The listing builds one solid part. Answer for the finished solid, in the listing's coordinates (mm). A direction names the side the tool comes from. Give positions to 0.01 mm unless a question says otherwise; leave off trailing zeros. Write each loop counter-clockwise with the first axis right and the second up, starting at its lowest first coordinate (ties: lowest second). Pieces come first, ordered by that corner, then holes. Notation, with made-up numbers: (54, 85) -> (65, 85) arc R21 cw to (65, 89) -> close; hole circle Ø2 at (27, 2). An arc over 180 degrees is marked (long way). Put each result on its own line as item: value. Start each with the question number.
1) A cutting plane is placed at D-D (y = 7.75). Write down the section's boundary in (x, z) (3 decimals), then the cut area to 3 significant figures.
2) For faces 4 (the flat face through (-11, 14, 8)), 5 (the flat face through (16.975, 2, -15)), 6 (the flat face through (-21, 26.1, 0)), 7 (the flat face through (26.175, 17, 0)), 8 (the flat face through (27, 5, -5)), determine the directions among +Z, -Z, +X, -X, +Y, -Y from which every point of the face is accessible in a straight line to the end or side of a thin tool.
3) A cutting plane is placed at B-B (y = 18.75). Write down the section's boundary in (x, z) (3 decimals), then the cut area to 3 significant figures.
4) A cutting plane is placed at C-C (z = -19.35). Write down the section's boundary in (x, y) (3 decimals), then the cut area to 3 significant figures.
5) Find the intervals of material crossed by line 1 along X through (y, z) = (2.7, 0) (3 decimals); line 2 along X through (y, z) = (3.1, 4) (3 decimals); line 3 along X through (y, z) = (3.9, -19.35) (3 decimals), in increasing order. Write a range as from..to.
6) For a pull along Y with two mould halves and no side action, classify faces 1 (the flat face through (-12, 5, 2.05)), 2 (the flat face through (39, 26.1, 0)), 3 (the cylindrical face through (22.737, 1.775, -0.347)) as released by +Y, released by -Y, zero draft, split by the parting line, or undercut.
7) A cutting plane is placed at A-A (y = 24.75). Write down the section's boundary in (x, z) (3 decimals), then the cut area to 3 significant figures.
8) Flat-ended cylindrical pins translate along their axes: pin 1 Ø15 at (x, y) = (-8, 12.5) entering from -Z; pin 2 Ø10 at (y, z) = (6.5, 0.5) entering from +X (3 decimals); pin 3 Ø10 at (x, z) = (-13.5, 2) entering from -Y; pin 4 Ø1 at (y, z) = (25, 6) entering from -X. Find the tip coordinate at first contact, or state that the pin passes through.
Autodesk Inventor part; units mm, degrees
ref_plane "YZ Plane" through (0, 0, 0) normal (1, 0, 0) x (0, 1, 0)
ref_plane "XZ Plane" through (0, 0, 0) normal (0, 1, 0) x (-1, 0, 0)
ref_plane "XY Plane" through (0, 0, 0) normal (0, 0, 1) x (1, 0, 0)
sketch "Эскиз1" plane through (0, 0, 0) normal (0, 1, 0) x (-1, 0, 0)
  line L0 (-8.725, 8) -> (8.725, 8)
  line L1 (8.725, 8) -> (8.725, -8)
  line L2 (8.725, -8) -> (-8.725, -8)
  line L3 (-8.725, -8) -> (-8.725, 8)
  line L4 (-8.725, 8) -> (8.725, -8) construction
  line L5 (8.725, 8) -> (-8.725, -8) construction
  point P0 (0, 0)
  dimension "d0" = 17.45
  dimension "d1" = 16
extrude "Выдавливание1" add sketch "Эскиз1" along normal blind 5
sketch "Эскиз2" plane through (-8.725, 0, -8) normal (-1, 0, 0) x (0, 0, 1)
  line L0 (0, 23.1) -> (16, 23.1)
  line L1 (16, 23.1) -> (16, 0)
  line L2 (16, 0) -> (0, 0)
  line L3 (0, 0) -> (0, 23.1)
  line L4 (16, 0) -> (16, 5)
  line L5 (0, 0) -> (0, 5)
  line L6 (0, 0) -> (16, 0)
  line L7 (0, 5) -> (16, 5)
  point P0 (8, 0)
  dimension "d5" = 18.1
extrude "Выдавливание2" add sketch "Эскиз2" along normal blind 5
sketch "Эскиз3" plane through (-8.725, 23.1, 8) normal (0, 1, 0) x (1, 0, 0)
  line L0 (0, 16) -> (-17.5, 16)
  line L1 (-17.5, 16) -> (-17.5, 0)
  line L2 (-17.5, 0) -> (0, 0)
  line L3 (0, 0) -> (0, 16)
  line L4 (0, 0) -> (-5, 0)
  circle A0 centre (-9.5, 8) radius 8
  line L5 (-5, 0) -> (-5, 16)
  point P0 (-9.5, 16)
  point P1 (-9.5, 0)
  point P2 (-5, 8)
  dimension "d49" = 4.5
extrude "Выдавливание3" add sketch "Эскиз3" along normal blind 6 contours L3 L2 L5 A0 L0 | L5 A0 L0 | A0 L5 | A0 L5 | L2 A0 L5
sketch "Эскиз7" plane through (0, 0, 0) normal (0, -1, 0) x (1, 0, 0)
  line L0 (-8.725, -8) -> (-8.725, 8) construction
  line L1 (-8.725, 8) -> (-8.725, -8) construction
  line L2 (-13.725, 8) -> (-13.725, -8) construction
  line L3 (-8.725, -8) -> (-13.725, -8) construction
  line L4 (-13.725, -8) -> (-13.725, 8) construction
  line L5 (-13.725, 8) -> (-8.725, 8) construction
  line L6 (-8.725, 8) -> (-8.725, -8) construction
  line L7 (-13.725, -8) -> (-13.725, 8)
  line L8 (-13.725, 0) -> (-8.725, 0) construction
  line L9 (-11.225, -4) -> (-11.225, 4)
  point P0 (0, 0)
  point P1 (-11.225, 0)
  dimension "d34" = 8
hole "Отверстие3" at (-11.225, 0, -4) at (-11.225, 0, 4) direction (0, 1, 0) diameter 2.2 depth 6
sketch "Эскиз8" plane through (0, 0, 0) normal (0, -1, 0) x (1, 0, 0)
  circle A0 centre (-11.225, -4) radius 1.1
  line L0 (-13.4767, -4) -> (-12.3508, -2.05) construction
  line L1 (-12.3508, -2.05) -> (-10.0992, -2.05)
  line L2 (-10.0992, -2.05) -> (-8.9733, -4)
  line L3 (-8.9733, -4) -> (-10.0992, -5.95)
  line L4 (-10.0992, -5.95) -> (-12.3508, -5.95)
  line L5 (-12.3508, -5.95) -> (-13.4767, -4) construction
  circle A1 centre (-11.225, 4) radius 1.1
  line L6 (-13.4767, 4) -> (-12.3508, 5.95) construction
  line L7 (-12.3508, 5.95) -> (-10.0992, 5.95)
  line L8 (-10.0992, 5.95) -> (-8.9733, 4)
  line L9 (-8.9733, 4) -> (-10.0992, 2.05)
  line L10 (-10.0992, 2.05) -> (-12.3508, 2.05)
  line L11 (-12.3508, 2.05) -> (-13.4767, 4) construction
  line L12 (-13.725, -8) -> (-13.725, 8)
  line L13 (-12.3508, -5.95) -> (-13.725, -5.95)
  line L14 (-13.725, -5.95) -> (-13.725, -2.05)
  line L15 (-13.725, -2.05) -> (-12.3508, -2.05)
  line L16 (-12.3508, -2.05) -> (-12.3508, -5.95) construction
  line L17 (-12.3508, 2.05) -> (-13.725, 2.05)
  line L18 (-13.725, 2.05) -> (-13.725, 5.95)
  line L19 (-13.725, 5.95) -> (-12.3508, 5.95)
  line L20 (-12.3508, 5.95) -> (-12.3508, 2.05) construction
  point P0 (0, 0)
  dimension "d42" = 3.9
extrude "Выдавливание5" cut sketch "Эскиз8" along normal blind 2.1 from surface at -6
sketch "Эскиз4" plane through (-8.725, 23.1, 8) normal (0, -1, 0) x (1, 0, 0)
  arc A0 (-9.5, 0) -> (-9.5, -16) centre (-9.5, -8) ccw
  circle A1 centre (-12.5, -8) radius 4
  arc A2 (-9.5, 0) -> (-9.5, -16) centre (-9.5, -8) ccw
  line L0 (-17.5, -8) -> (-16.5, -8) construction
  line L1 (-16.5, -8) -> (-9.5, -8) construction
  point P0 (8.725, -8)
  dimension "d45" = 8
  dimension "d46" = 1
extrude "Выдавливание6" cut sketch "Эскиз4" against normal blind 3
sketch "Эскиз5" plane through (0, 5, 0) normal (0, 1, 0) x (1, 0, 0)
  line L0 (-8.725, 8) -> (-8.725, -8)
  line L1 (-8.725, 0) -> (-3.725, 0) construction
  point P0 (0, 0)
  dimension "d22" = 5
hole "Отверстие2" at (-3.725, 5, 0) direction (0, -1, 0) diameter 3.2 end through all countersink diameter 6 countersink angle 90
mirror "Зеркальное отражение1" about plane through (8.725, 0, 8) normal (1, 0, 0)
sketch "Эскиз9" plane through (0, 0, 0) normal (0, -1, 0) x (1, 0, 0)
  line L0 (-8.725, 8) -> (26.175, 8) construction
  line L1 (8.725, 8) -> (8.725, -8) construction
  line L2 (-8.725, -8) -> (26.175, -8) construction
  line L3 (2.475, -16.35) -> (14.975, -16.35) construction
  line L4 (14.975, -16.35) -> (14.975, 6.45) construction
  line L5 (14.975, 6.45) -> (2.475, 6.45) construction
  line L6 (2.475, 6.45) -> (2.475, -16.35) construction
  line L7 (2.475, -16.35) -> (14.975, 6.45) construction
  line L8 (14.975, -16.35) -> (2.475, 6.45) construction
  line L9 (16.975, 10.95) -> (0.475, 10.95)
  line L10 (0.475, 10.95) -> (0.475, -22.35)
  line L11 (0.475, -22.35) -> (16.975, -22.35)
  line L12 (16.975, -22.35) -> (16.975, 10.95)
  point P0 (0, 0)
  point P1 (8.725, -4.95)
  point P2 (8.725, 0)
  dimension "d50" = 12.5
  dimension "d51" = 22.8
  dimension "d59" = 4.95
  dimension "d68" = 6
  dimension "d69" = 4.5
  dimension "d70" = 2
  dimension "d71" = 2
extrude "Выдавливание7" add sketch "Эскиз9" against normal up to surface (5 mm away)
sketch "Эскиз10" plane through (0, 5, 0) normal (0, 1, 0) x (1, 0, 0)
  line L0 (2.275, -6.45) -> (15.175, -6.45)
  line L1 (15.175, -6.45) -> (15.175, 16.35)
  line L2 (15.175, 16.35) -> (2.275, 16.35)
  line L3 (2.275, 16.35) -> (2.275, -6.45)
  line L4 (2.275, -6.45) -> (15.175, 16.35) construction
  line L5 (15.175, -6.45) -> (2.275, 16.35) construction
  line L6 (-8.725, 8) -> (0.475, 8)
  line L7 (16.975, -8) -> (0.475, 8) construction
  line L8 (16.975, 8) -> (26.175, 8)
  line L9 (-8.725, -8) -> (0.475, -8)
  line L10 (16.975, 8) -> (0.475, -8) construction
  line L11 (16.975, -8) -> (26.175, -8)
  line L12 (8.725, 0) -> (8.725, 4.95)
  point P0 (0, 0)
  dimension "d54" = 12.9
  dimension "d55" = 22.8
  dimension "d72" = 4.95
extrude "Выдавливание8" cut sketch "Эскиз10" against normal through all
sketch "Эскиз11" plane through (0, 0, 0) normal (0, -1, 0) x (1, 0, 0)
  line L0 (8.725, -22.35) -> (8.725, -16.35) construction
  line L1 (12.725, -19.35) -> (4.725, -19.35)
  line L2 (15.175, -16.35) -> (2.275, -16.35)
  line L3 (0.475, -22.35) -> (16.975, -22.35)
  point P0 (0, 0)
  point P1 (8.725, -19.35)
  dimension "d60" = 8
hole "Отверстие4" at (12.725, 0, -19.35) at (4.725, 0, -19.35) direction (0, 1, 0) diameter 2.2 end through all countersink diameter 4.2 countersink angle 90
sketch "Эскиз12" plane through (0, 5, 0) normal (0, 1, 0) x (1, 0, 0)
  line L0 (2.275, -6.45) -> (15.175, -6.45)
  line L1 (15.175, -6.45) -> (2.275, -6.45)
  line L2 (2.275, -6.45) -> (2.275, -10.95)
  line L3 (2.275, -10.95) -> (15.175, -10.95)
  line L4 (15.175, -10.95) -> (15.175, -6.45)
  line L5 (16.975, -10.95) -> (0.475, -10.95)
  point P0 (0, 0)
extrude "Выдавливание9" add sketch "Эскиз12" along normal blind 10.6
sketch "Эскиз13" plane through (0, 15.6, 0) normal (0, 1, 0) x (1, 0, 0)
  line L0 (8.725, -8.525) -> (8.725, -6.45) construction
  line L1 (2.275, -6.45) -> (15.175, -6.45)
  point P0 (0, 0)
  dimension "d82" = 2.075
hole "Отверстие5" at (8.725, 15.6, 8.525) direction (0, -1, 0) diameter 2 depth 6000 tip angle 118
properties part number "Basis of steering"
Reply:
1. outline: (-13.725, -8) -> (-8.725, -8) -> (-8.725, 8) -> (-13.725, 8) -> close; (2.275, 6.45) -> (15.175, 6.45) -> (15.175, 10.95) -> (2.275, 10.95) -> close; (26.175, -8) -> (31.175, -8) -> (31.175, 8) -> (26.175, 8) -> close; hole circle Ø2 at (8.725, 8.525)
1. area: 215 mm2
2. face 4: +Z, -X, +Y, -Y
2. face 5: -Z, +X, +Y, -Y
2. face 6: -Y
2. face 7: +Z, -Z, +Y
2. face 8: +X
3. outline: (-13.725, -8) -> (-8.725, -8) -> (-8.725, 8) -> (-13.725, 8) -> close; (26.175, -8) -> (31.175, -8) -> (31.175, 8) -> (26.175, 8) -> close
3. area: 160 mm2
4. outline: (0.475, 0) -> (2.625, 0) -> (3.625, 1) -> (3.625, 5) -> (0.475, 5) -> close; (5.825, 1) -> (6.825, 0) -> (10.625, 0) -> (11.625, 1) -> (11.625, 5) -> (5.825, 5) -> close; (13.825, 1) -> (14.825, 0) -> (16.975, 0) -> (16.975, 5) -> (13.825, 5) -> close
4. area: 58.5 mm2
5. line 1: x = -13.725..-5.325, -2.125..2.275, 15.175..19.575, 22.775..31.175
5. line 2: x = -13.725..-12.325, -10.125..2.275, 15.175..27.575, 29.775..31.175
5. line 3: x = 0.475..3.625, 5.825..11.625, 13.825..16.975
6. face 1: undercut
6. face 2: released by -Y
6. face 3: zero draft
7. outline: (-18.225, -8) -> (-8.725, -8) -> (-8.725, 8) -> (-18.225, 8) arc R8 ccw to start; (26.175, -8) -> (35.675, -8) arc R8 ccw to (35.675, 8) -> (26.175, 8) -> close; hole circle Ø8 at (-21.225, 0); hole circle Ø8 at (38.675, 0)
7. area: 405 mm2
8. pin 1: stops at z = -8
8. pin 2: stops at x = 31.175
8. pin 3: stops at y = 0
8. pin 4: stops at x = -24.03
